Source: CAD feature listing. Evaluate the final solid. Frame: model axes, mm. A direction names the side the tool comes from. Coordinates: 2 decimals unless noted, no trailing zeros. Order: outer loops, then holes, each group sorted by start corner. A loop starts at its lowest first (then second) coordinate and runs counter-clockwise, first axis right, second up. Notation, with made-up numbers: (-23.5, 56.5) - (-1.5, 56.5) arc R24 ccw to (-1.5, 86.5) - close; hole circle Ø8 at (-17.5, 13.25). An arc over 180 degrees is marked (long way). One line per question, with ' | ' between items.
from build123d import *

# Parameters (mm, degrees)
CYLINDER_R        = 1.6
CYLINDER_DEPTH    = 10
BOX001_W          = 12
BOX001_H          = 12
BOX001_DEPTH      = 1
BOX_W             = 30
BOX_H             = 12
BOX_DEPTH         = 3
CYLINDER001_R     = 1.6
CYLINDER001_DEPTH = 10


with BuildPart() as cylinder:
    # Cylinder → Cylinder (new body)
    with BuildSketch(Plane(origin=(25.5, 6, -7), x_dir=(1, 0, 0), z_dir=(0, 0, 1))):
        Circle(CYLINDER_R)
    extrude(amount=CYLINDER_DEPTH)


with BuildPart() as obj1:
    # Box001 → Box001 (new body)
    with BuildSketch(Plane(origin=(9, 0, 2), x_dir=(1, 0, 0), z_dir=(0, 0, 1))):
        with Locations((6, 6)):
            Rectangle(BOX001_W, BOX001_H)
    extrude(amount=BOX001_DEPTH)


with BuildPart() as fusion:
    # Box → Box (new body)
    with BuildSketch(Plane.XY):
        with Locations((15, 6)):
            Rectangle(BOX_W, BOX_H)
    extrude(amount=BOX_DEPTH)

    # Cut: cut obj1
    add(obj1.part, mode=Mode.SUBTRACT)

    # Fusion: union Cylinder
    add(cylinder.part)


with BuildPart() as obj2:
    # Cylinder001 → Cylinder001 (new body)
    with BuildSketch(Plane(origin=(4.5, 6, -7), x_dir=(1, 0, 0), z_dir=(0, 0, 1))):
        Circle(CYLINDER001_R)
    extrude(amount=CYLINDER001_DEPTH)

    # Fusion001: union Fusion
    add(fusion.part)


solid = obj2.part
(1) Cut plane C-C (z = -5). Return the cut outline in (x, y), and give its area (3 significant figures).
Taken from the geometry:
outline: circle Ø3.2 at (4.5, 6); circle Ø3.2 at (25.5, 6) | area: 16.1 mm²
(2) Pull-direction query (X, two-part tool) for faces 4 (the flat face through (0, 6, 1)), 5 (the cylindrical face through (4.15, 4.44, -3.55)), 6 (the flat face through (25, 6, 3)); classes: pulls with the +X half, pulls with the -X half, needs draft (parallel to the pull), parting line crosses it, or undercut.
Taken from the geometry:
face 4: pulls with the -X half | face 5: undercut | face 6: needs draft
(3) Cut plane B-B (x = 25.5). Return the cut outline in (y, z).
Taken from the geometry:
outline: (0, 0) - (4.4, 0) - (4.4, -7) - (7.6, -7) - (7.6, 0) - (12, 0) - (12, 3) - (0, 3) - close
(4) Cut plane A-A (y = 9.5). Return the cut outline in (x, z), and give its area (3 significant figures).
Taken from the geometry:
outline: (0, 0) - (30, 0) - (30, 3) - (21, 3) - (21, 2) - (9, 2) - (9, 3) - (0, 3) - close | area: 78.0 mm²
(5) Material intervals for L1, parallel to X at y = 10, z = 2.75; L2, parallel to Z at x = 5.5, y = 8.5; L3, parallel to Z at x = 13.25, y = 5.75, sorted ascending. Write a range as from..to.
Taken from the geometry:
L1: x = 0..9, 21..30 | L2: z = 0..3 | L3: z = 0..2
(6) Cut plane D-D (y = 6). Return the cut outline in (x, z), and give its area (3 significant figures).
Taken from the geometry:
outline: (0, 0) - (2.9, 0) - (2.9, -7) - (6.1, -7) - (6.1, 0) - (23.9, 0) - (23.9, -7) - (27.1, -7) - (27.1, 0) - (30, 0) - (30, 3) - (21, 3) - (21, 2) - (9, 2) - (9, 3) - (0, 3) - close | area: 123 mm²
(7) Set-up query: faces 1 (the cylindrical face through (25.15, 4.44, -3.55)), 2 (the flat face through (15, 6, 2)), 3 (the flat face through (25, 6, -7)). Return all of +Z, -Z, +X, -X, +Y, -Y with unobstructed straight access to the full face (end or side cutting, diameter ignored); none if empty.
Taken from the geometry:
face 1: -Z | face 2: +Z, +Y, -Y | face 3: -Z, +X, -X, +Y, -Y
